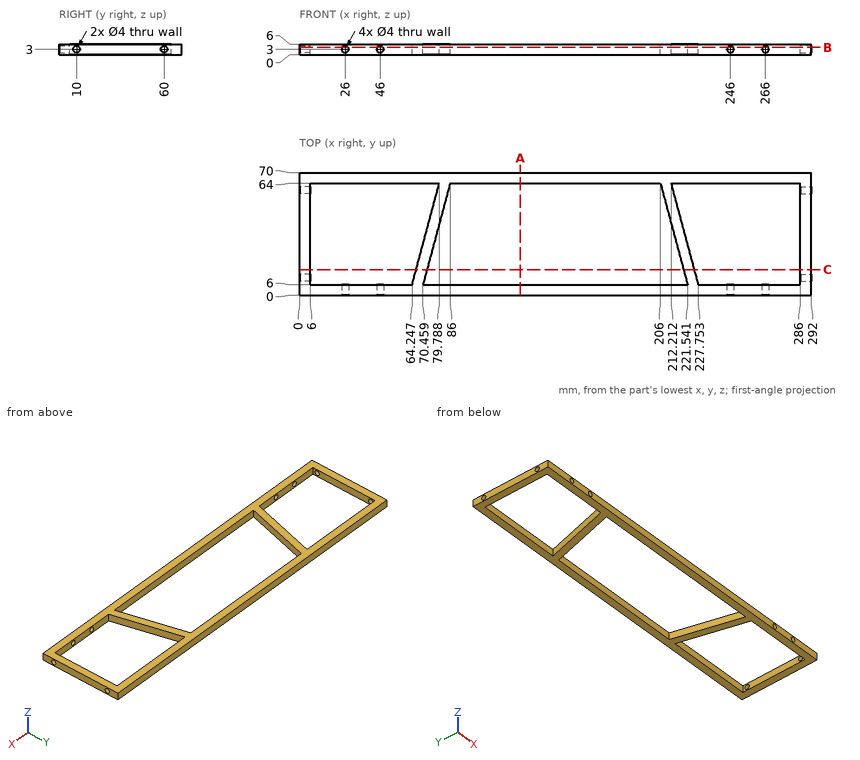
Here's the drawing with two shaded views (mm, measured from the low corner). I have some questions. Give positions to 0.01 mm unless a question says otherwise; leave off trailing zeros. Order: outer loops, then holes, each group sorted by start corner. A loop starts at its lowest first (then second) coordinate and runs counter-clockwise, first axis right, second up. Notation, with made-up numbers: M 67,86 L 123,86 A25 cw 123,100 Z; hole C 45.25,16 d11. An arc over 180 degrees is marked long. One line per item, written item: value.
1) I want a section at C-C, the plane y = 14.5. List the corners of the cut face in (x, z) for me (1 decimal).
Answer sheet:
outline: M 0,0 L 6,0 L 6,6 L 0,6 Z; M 66.5,0 L 72.7,0 L 72.7,6 L 66.5,6 Z; M 219.3,0 L 225.5,0 L 225.5,6 L 219.3,6 Z; M 286,0 L 292,0 L 292,6 L 286,6 Z
2) I want a section at A-A, the plane x = 126. List the corners of the cut face in (y, z) for me.
Answer sheet:
outline: M 0,0 L 6,0 L 6,6 L 0,6 Z; M 64,0 L 70,0 L 70,6 L 64,6 Z
3) For P1, Ø3.5, axis at x = 266, z = 3, coming from the -Y side, with a flat end and sliding along its axis, tell me the tip position at first contact or that it passes through.
Answer sheet:
P1: stops at y = 64
4) I want a section at B-B, the plane z = 4.1. Count the separate pieces of the cut face and the enclosed holes in it, plus the area to 3 significant figures.
Answer sheet:
separate pieces: 7
enclosed holes: 1
area: 4,760 mm^2
5) Please list where these lines run through material, in increasing order: line 1 along Y through (x, z) = (290.7, 3); line 2 along X through (y, z) = (2.2, 3); line 3 along Y through (x, z) = (24.5, 1.5).
Answer sheet:
line 1: y = 0 to 8, 12 to 58, 62 to 70
line 2: x = 0 to 24, 28 to 44, 48 to 244, 248 to 264, 268 to 292
line 3: y = 0 to 6, 64 to 70
